For this review, take the finished solid that the model builds, in its own axes (mm). Face numbers are marked on the shaded views. A direction names the side the tool comes from. Round coordinates to 2 decimals unless told otherwise and drop trailing zeros. Order: outer loops, then holes, each group sorted by start corner. A loop starts at its lowest first (then second) coordinate and runs counter-clockwise, first axis right, second up. Notation, with made-up numbers: (-21.75, 34.25) -> (18.25, 34.25) arc R18 cw to (18.25, 66.25) -> close; hole circle Ø5 at (68, 25). An arc over 180 degrees is marked (long way). Use a Markdown table: item, result. Add a question column.
1) Consider section A-A (z = 46.5). State the section outline as (x, y) points, plus the area to 3 significant figures.
2) Consider section B-B (z = 97). State the section outline as (x, y) points.
3) Clearance check with flat-ended pins moving along their axes: P1, Ø5, axis at x = -97, y = -93, coming from the -Z side; P2, Ø12, axis at y = 56.5, z = 134.5, coming from the +X side; P3, Ø4, axis at x = 131, y = 18.5, coming from the +Z side. State where each tip first meets the part, or that it passes through.
4) Machinability: for the marked faces 1 and 2, which of the approach directions +Z, -Z, +X, -X, +Y, -Y give a long, thin tool a straight path to every point of the face, cutting with its end or side? Answer none if there is none.
5) Draft analysis for pull direction X (two halves, no side actions). For the marked faces 3, 4 and 5, state which applies: pulls with the +X half, pulls with the -X half, needs draft (parallel to the pull), parting line crosses it, or undercut.
6) Wall thickness on line 1 along Y through (x, z) = (0, 187); line 2 along Z through (x, y) = (12.5, -8): over which ranges is each line inside the solid? List them lowest first. Write a range as [from, to].
```python
from build123d import *

# Parameters (mm, degrees)
F2_R = 20
F3_R = 30
F4_R = 40


with BuildPart() as f1:
    # F0 (on Front) → F1 (revolve)
    with BuildSketch(Plane.XZ):
        Polygon((0, 216), (0, 198), (45, 198), (45, 157.226497), (185.301924, 76.223143), (172, 0), (177, 0), (198, 80.438912), (55, 163), (55, 216), align=None)
    revolve(axis=Axis((0, 0, 99), (0, 0, 1)))

    # F2
    f2_edges = [f1.edges().sort_by_distance(p)[0] for p in [
        (-185.301924, 0, 76.223143),
    ]]
    fillet(f2_edges, radius=F2_R)

    # F3
    f3_edges = [f1.edges().sort_by_distance(p)[0] for p in [
        (-198, 0, 80.438912),
        (-55, 0, 163),
    ]]
    fillet(f3_edges, radius=F3_R)

    # F4
    f4_edges = [f1.edges().sort_by_distance(p)[0] for p in [
        (-45, 0, 157.226497),
    ]]
    fillet(f4_edges, radius=F4_R)


solid = f1.part
```
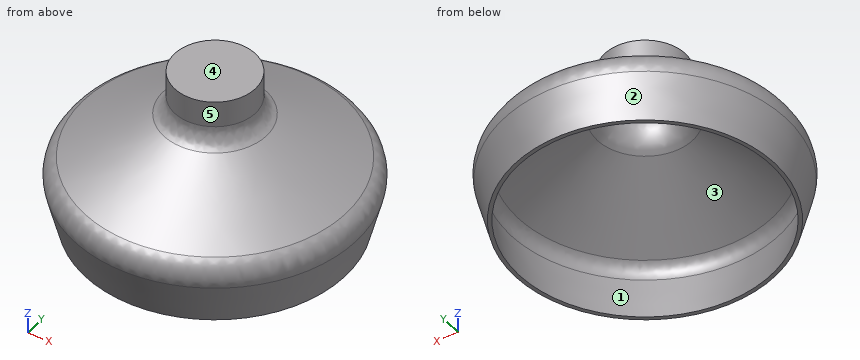
Results list:
| question | item | result |
|---|---|---|
| 1 | outline | circle Ø378.28 at (0, 0); hole circle Ø360.23 at (0, 0) |
| 1 | area | 10,500 mm2 |
| 2 | outline | circle Ø338.63 at (0, 0); hole circle Ø298.63 at (0, 0) |
| 3 | P1 | z = 104.18 |
| 3 | P2 | x = 100.34 |
| 3 | P3 | z = 119.53 |
| 4 | face 1 | none |
| 4 | face 2 | -Z |
| 5 | face 3 | undercut |
| 5 | face 4 | needs draft |
| 5 | face 5 | parting line crosses it |
| 6 | line 1 | [-55, -45], [45, 55] |
| 6 | line 2 | [198, 216] |
